Part model, mm, in its own coordinate system. A direction names the side the tool comes from. Round coordinates to 2 decimals unless told otherwise and drop trailing zeros. Loops run counter-clockwise (first coordinate to the right, second up) from the corner with the lowest first, then second, coordinate; pieces in that order, holes last. Notation, with made-up numbers: (-20, 78) - (24, 78) arc R13 cw to (24, 87) - close; hole circle Ø9 at (21, -14.5). An arc over 180 degrees is marked (long way). Put each result on its own line as item: value.
from build123d import *

# Parameters (mm, degrees)
SKETCH_1_W             = 12.5
SKETCH_1_H             = 50
EXTRUDE_1_DEPTH        = 34
SKETCH_2_R             = 7.5
CUT_EXTRUDE_1_DEPTH    = 13.25
CUT_EXTRUDE_START      = -13.5
SKETCH_3_R             = 1.65
CUT_EXTRUDE_2_DEPTH    = 14.5
SKETCH_4_R             = 2.9
CUT_EXTRUDE_3_DEPTH    = 4.5
SKETCH_5_R             = 5.5
CUT_EXTRUDE_4_DEPTH    = 35
EXTRUDE_2_DEPTH        = 17
SKETCH_9_R             = 1.65
CUT_EXTRUDE_6_DEPTH    = 6
CUT_EXTRUDE_5_DEPTH    = 9
PATTERN_LINEAR_1_COUNT = 2
PATTERN_LINEAR_1_PITCH = 24


with BuildPart() as part:
    # 草图1 → 凸台-拉伸1 (new body)
    with BuildSketch(Plane(origin=(0, 0, 0), x_dir=(0, 0, -1), z_dir=(1, 0, 0))):
        with Locations((6.25, 25)):
            Rectangle(SKETCH_1_W, SKETCH_1_H)
    extrude(amount=EXTRUDE_1_DEPTH)

    # 草图2 → 切除-拉伸1 (cut, symmetric)
    with BuildSketch(Plane.ZY.offset(-17)):
        with Locations((0, 18)):
            Circle(SKETCH_2_R)
        with Locations((0, 42)):
            Circle(SKETCH_2_R)
    extrude(amount=CUT_EXTRUDE_1_DEPTH, both=True, mode=Mode.SUBTRACT)

    # 草图3 → 切除-拉伸2 (cut)
    with BuildSketch(Plane(origin=(0, 0, -12.5), x_dir=(-1, 0, 0), z_dir=(0, 0, -1)).offset(CUT_EXTRUDE_START)):
        with Locations((-29, 30)):
            Circle(SKETCH_3_R)
        with Locations((-5, 30)):
            Circle(SKETCH_3_R)
        with Locations((-17, 30)):
            Circle(SKETCH_3_R)
    cut_extrude_2 = extrude(amount=CUT_EXTRUDE_2_DEPTH, mode=Mode.SUBTRACT)

    # 草图4 → 切除-拉伸3 (cut)
    with BuildSketch(Plane(origin=(0, 0, -12.5), x_dir=(-1, 0, 0), z_dir=(0, 0, -1))):
        with Locations((-29, 30)):
            Circle(SKETCH_4_R)
        with Locations((-5, 30)):
            Circle(SKETCH_4_R)
    extrude(amount=-CUT_EXTRUDE_3_DEPTH, mode=Mode.SUBTRACT)

    # 草图5 → 切除-拉伸4 (cut, through all)
    with BuildSketch(Plane(origin=(34, 0, 0), x_dir=(0, 0, -1), z_dir=(1, 0, 0))):
        with Locations((0, 18)):
            Circle(SKETCH_5_R)
        with Locations((0, 42)):
            Circle(SKETCH_5_R)
    extrude(amount=-CUT_EXTRUDE_4_DEPTH, mode=Mode.SUBTRACT)

    # 草图6 → 凸台-拉伸2 (add, symmetric)
    with BuildSketch(Plane.ZY.offset(-17)):
        Polygon((-12.5, 50), (-17.5, 50), (-17.5, 45), (-12.5, 40), align=None)
    extrude(amount=EXTRUDE_2_DEPTH, both=True)

    # 草图9 → 切除-拉伸6 (cut, through all)
    with BuildSketch(Plane(origin=(0, 45, 0), x_dir=(1, 0, 0), z_dir=(0, 1, 0))):
        with Locations((5, 12)):
            Circle(SKETCH_9_R)
        with Locations((17, 12)):
            Circle(SKETCH_9_R)
        with Locations((29, 12)):
            Circle(SKETCH_9_R)
    extrude(amount=CUT_EXTRUDE_6_DEPTH, mode=Mode.SUBTRACT)

    # 草图7 → 切除-拉伸5 (cut)
    with BuildSketch(Plane(origin=(0, 45, 0), x_dir=(1, 0, 0), z_dir=(0, 1, 0))):
        Polygon((7.85, 10.354551733), (7.85, 13.090838694), (7.85, 17.5), (2.15, 17.5), (2.15, 12.981963635), (2.15, 10.354551733), (5, 8.709103466), align=None)
        Polygon((19.85, 10.354551733), (19.85, 13.090959175), (19.85, 17.5), (14.15, 17.5), (14.15, 12.981963635), (14.15, 10.354551733), (17, 8.709103466), align=None)
        Polygon((31.85, 10.354551733), (31.85, 13.090958614), (31.85, 17.5), (26.15, 17.5), (26.15, 12.981963635), (26.15, 10.354551733), (29, 8.709103466), align=None)
    extrude(amount=-CUT_EXTRUDE_5_DEPTH, mode=Mode.SUBTRACT)

    # 阵列(线性)1: 切除-拉伸2 ×2
    with Locations(*[(0, -i * PATTERN_LINEAR_1_PITCH, 0) for i in range(1, PATTERN_LINEAR_1_COUNT)]):
        add(cut_extrude_2, mode=Mode.SUBTRACT)


solid = part.part
1. Band-saw the part on A-A (y = 30). List the corners of the cut face in (x, z).
A:
outline: (0, -12.5) - (2.1, -12.5) - (2.1, -8) - (3.35, -8) - (3.35, 0) - (0, 0) - close; (6.65, -8) - (7.9, -8) - (7.9, -12.5) - (15.35, -12.5) - (15.35, 0) - (6.65, 0) - close; (18.65, -12.5) - (26.1, -12.5) - (26.1, -8) - (27.35, -8) - (27.35, 0) - (18.65, 0) - close; (30.65, -8) - (31.9, -8) - (31.9, -12.5) - (34, -12.5) - (34, 0) - (30.65, 0) - close
2. Band-saw the part on B-B (z = -1). Give the number of separate pieces and of enclosed holes in the cut face, plus the area to 3 significant figures.
A:
separate pieces: 3
enclosed holes: 6
area: 699 mm²
3. Probe line 1 along Y through (x, z) = (17, -9.25); line 2 along X through (y, z) = (6, -8); line 3 along X through (y, z) = (19, -6). List the from-to ranges inside material, lowest first. Write a range as [from, to].
A:
line 1: y = [0, 4.35], [7.65, 28.35], [31.65, 36], [45, 50]
line 2: x = [0, 3.35], [6.65, 15.35], [18.65, 27.35], [30.65, 34]
line 3: x = [0, 3.75], [30.25, 34]
4. Band-saw the part on C-C (z = -14.5). List the corners of the cut face in (x, y), plus the area to 3 significant figures.
A:
outline: (0, 42) - (2.15, 42) - (2.15, 45) - (7.85, 45) - (7.85, 42) - (14.15, 42) - (14.15, 45) - (19.85, 45) - (19.85, 42) - (26.15, 42) - (26.15, 45) - (31.85, 45) - (31.85, 42) - (34, 42) - (34, 50) - (0, 50) - close
area: 221 mm²
5. Two-plate mould, pull along X, no slides. Class faces 4 (the cylindrical face through (1.9, 17.9, -5.5)), 5 (the flat face through (27.56, 40.56, -9.54)), 6 (the flat face through (34, 25, -7)): pulls with the +X half, pulls with the -X half, needs draft (parallel to the pull), parting line crosses it, or undercut.
A:
face 4: needs draft
face 5: undercut
face 6: pulls with the +X half
6. Pin check, flat tips, straight feed: P1, Ø2, axis at x = 29, z = -12, coming from the +Y side; P2, Ø3, axis at x = 29.5, y = 30.5, coming from the -Z side; P3, Ø1, axis at x = 24, z = -14.5, coming from the -Y side. Stop position of each tip, or through.
A:
P1: stops at y = 36
P2: stops at z = -8
P3: stops at y = 41.5
7. Tool access for faces 1 (the flat face through (30.25, 19.8, -5.5)), 2 (the flat face through (26.15, 42, -12)), 3 (the cylindrical face through (27.69, 47.46, -11)): list every direction of +Z, -Z, +X, -X, +Y, -Y with a clear straight run to the whole face (end or side of a thin tool).
A:
face 1: +Z
face 2: -Z
face 3: +Y
8. Band-saw the part on D-D (y = 42). List the corners of the cut face in (x, z).
A:
outline: (0, -14.5) - (2.15, -14.5) - (2.15, -10.35) - (5, -8.71) - (7.85, -10.35) - (7.85, -14.5) - (14.15, -14.5) - (14.15, -10.35) - (17, -8.71) - (19.85, -10.35) - (19.85, -14.5) - (26.15, -14.5) - (26.15, -10.35) - (29, -8.71) - (31.85, -10.35) - (31.85, -14.5) - (34, -14.5) - (34, -5.5) - (30.25, -5.5) - (30.25, -7.5) - (3.75, -7.5) - (3.75, -5.5) - (0, -5.5) - close
